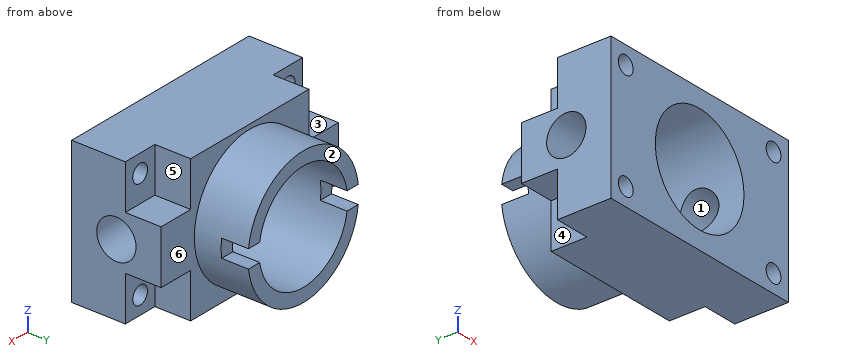
from build123d import *

# Parameters (mm, degrees)
SKETCH_1_W          = 120
SKETCH_1_H          = 80
EXTRUDE_1_DEPTH     = 50
SKETCH_2_W          = 20
SKETCH_2_H          = 25
CUT_EXTRUDE_1_DEPTH = 20
SKETCH_3_R          = 5
CUT_EXTRUDE_2_DEPTH = 30
SKETCH_5_R          = 11
CUT_EXTRUDE_4_DEPTH = 120
SKETCH_6_R          = 37.5
EXTRUDE_2_DEPTH     = 30
SKETCH_7_R          = 30
CUT_EXTRUDE_5_DEPTH = 81
CUT_EXTRUDE_6_DEPTH = 15


with BuildPart() as part:
    # Эскиз1 → Бобышка-Вытянуть1 (new body)
    with BuildSketch(Plane(origin=(0, 0, 0), x_dir=(1, 0, 0), z_dir=(0, 1, 0))):
        Rectangle(SKETCH_1_W, SKETCH_1_H)
    extrude(amount=EXTRUDE_1_DEPTH)

    # Эскиз2 → Вырез-Вытянуть1 (cut)
    with BuildSketch(Plane(origin=(0, 50, 0), x_dir=(1, 0, 0), z_dir=(0, 1, 0))):
        with Locations((-50, 27.5)):
            Rectangle(SKETCH_2_W, SKETCH_2_H)
        with Locations((-50, -27.5)):
            Rectangle(SKETCH_2_W, SKETCH_2_H)
        with Locations((50, -27.5)):
            Rectangle(SKETCH_2_W, SKETCH_2_H)
        with Locations((50, 27.5)):
            Rectangle(SKETCH_2_W, SKETCH_2_H)
    extrude(amount=-CUT_EXTRUDE_1_DEPTH, mode=Mode.SUBTRACT)

    # Эскиз3 → Вырез-Вытянуть2 (cut)
    with BuildSketch(Plane(origin=(0, 30, 0), x_dir=(1, 0, 0), z_dir=(0, 1, 0))):
        with Locations((-50, -30)):
            Circle(SKETCH_3_R)
        with Locations((-50, 30)):
            Circle(SKETCH_3_R)
        with Locations((50, 30)):
            Circle(SKETCH_3_R)
        with Locations((50, -30)):
            Circle(SKETCH_3_R)
    extrude(amount=-CUT_EXTRUDE_2_DEPTH, mode=Mode.SUBTRACT)

    # Эскиз5 → Вырез-Вытянуть4 (cut)
    with BuildSketch(Plane.ZY.offset(60)):
        with Locations((0, 25)):
            Circle(SKETCH_5_R)
    extrude(amount=-CUT_EXTRUDE_4_DEPTH, mode=Mode.SUBTRACT)

    # Эскиз6 → Бобышка-Вытянуть2 (add)
    with BuildSketch(Plane(origin=(0, 50, 0), x_dir=(1, 0, 0), z_dir=(0, 1, 0))):
        Circle(SKETCH_6_R)
    extrude(amount=EXTRUDE_2_DEPTH)

    # Эскиз7 → Вырез-Вытянуть5 (cut, through all)
    with BuildSketch(Plane(origin=(0, 80, 0), x_dir=(1, 0, 0), z_dir=(0, 1, 0))):
        Circle(SKETCH_7_R)
    extrude(amount=-CUT_EXTRUDE_5_DEPTH, mode=Mode.SUBTRACT)

    # Эскиз8 → Вырез-Вытянуть6 (cut)
    with BuildSketch(Plane(origin=(0, 80, 0), x_dir=(1, 0, 0), z_dir=(0, 1, 0))):
        with BuildLine():
            Line((-29.580398915, -5), (-37.165171868, -5))
            ThreePointArc((-37.165171868, -5), (-37.5, 0), (-37.165171868, 5))
            Line((-37.165171868, 5), (-29.580398915, 5))
            ThreePointArc((-29.580398915, 5), (-30, 0), (-29.580398915, -5))
        make_face()
        with BuildLine():
            Line((37.165171868, 5), (29.580398915, 5))
            ThreePointArc((29.580398915, 5), (30, 0), (29.580398915, -5))
            Line((29.580398915, -5), (37.165171868, -5))
            ThreePointArc((37.165171868, -5), (37.5, 0), (37.165171868, 5))
        make_face()
    extrude(amount=-CUT_EXTRUDE_6_DEPTH, mode=Mode.SUBTRACT)


solid = part.part
Model file for the job. Use its own axes, mm. Face numbers are marked on the shaded views. A direction names the side the tool comes from. Give positions to 0.01 mm unless a question says otherwise; leave off trailing zeros. Loops run counter-clockwise (first coordinate to the right, second up) from the corner with the lowest first, then second, coordinate; pieces in that order, holes last. Notation, with made-up numbers: (2, 87.5) -> (11, 87.5) arc R18 ccw to (11, 113.5) -> close; hole circle Ø8 at (45.5, 28.25). An arc over 180 degrees is marked (long way). Use a Markdown table: item, result. Add a question column.
(1) Slice it at D-D on x = 0. List the corners of the cut face in (y, z), and give its area (3 significant figures).
(2) Slice it at A-A on x = 50. List the corners of the cut face in (y, z), and give its area (3 significant figures).
(3) Tool access for the marked faces 4, 5 and 6: list every direction of +Z, -Z, +X, -X, +Y, -Y with a clear straight run to the whole face (end or side of a thin tool).
(4) Wall check: line 1 along X through (y, z) = (29.5, -30.5); line 2 along Z through (x, y) = (-54, 16.5); line 3 along Z through (x, y) = (50, 19.75). Give the ranges that are in metal, low to high.
(5) Slice it at B-B on y = 25. List the corners of the cut face in (x, z), and give its area (3 significant figures).
(6) Mould opens along Y. For the marked faces 1, 2 and 3 say: +Y half, -Y half, draft (parallel to the pull), parting line (faces both ways), or undercut.
(7) Slice it at C-C on z = 19. List the corners of the cut face in (x, y).
(8) Drop flat-ended pins along their axis: pin 1 Ø1.5 at (x, z) = (-24.5, -15.5) entering from -Y; pin 2 Ø8.5 at (x, y) = (32, 73) entering from +Z; pin 3 Ø22 at (x, y) = (55, 37.5) entering from -Z; pin 4 Ø2.5 at (x, z) = (34.5, 0.5) entering from +Y. Give the stop position or say it passes through.
Filled sheet:
| question | item | result |
|---|---|---|
| 1 | outline | (0, -40) -> (50, -40) -> (50, -37.5) -> (80, -37.5) -> (80, -30) -> (0, -30) -> close; (0, 30) -> (80, 30) -> (80, 37.5) -> (50, 37.5) -> (50, 40) -> (0, 40) -> close |
| 1 | area | 1,450 mm2 |
| 2 | outline | (0, -40) -> (30, -40) -> (30, -35) -> (0, -35) -> close; (0, -25) -> (30, -25) -> (30, -15) -> (50, -15) -> (50, 15) -> (30, 15) -> (30, 25) -> (0, 25) -> close; (0, 35) -> (30, 35) -> (30, 40) -> (0, 40) -> close; hole circle Ø22 at (25, 0) |
| 2 | area | 2,020 mm2 |
| 3 | face 4 | -Z, -X, +Y |
| 3 | face 5 | +Z, +X, +Y |
| 3 | face 6 | +Y |
| 4 | line 1 | -60 to -54.97, -45.03 to 45.03, 54.97 to 60 |
| 4 | line 2 | -40 to -33, -27 to -6.98, 6.98 to 27, 33 to 40 |
| 4 | line 3 | -40 to -35, -25 to -9.67, 9.67 to 25, 35 to 40 |
| 5 | outline | (-60, -40) -> (60, -40) -> (60, -11) -> (27.91, -11) arc R30 cw to (-27.91, -11) -> (-60, -11) -> close; (-60, 11) -> (-27.91, 11) arc R30 cw to (27.91, 11) -> (60, 11) -> (60, 40) -> (-60, 40) -> close; hole circle Ø10 at (-50, -30); hole circle Ø10 at (-50, 30); hole circle Ø10 at (50, -30); hole circle Ø10 at (50, 30) |
| 5 | area | 5,110 mm2 |
| 6 | face 1 | undercut |
| 6 | face 2 | +Y half |
| 6 | face 3 | draft |
| 7 | outline | (-60, 0) -> (-23.22, 0) -> (-23.22, 80) -> (-32.33, 80) -> (-32.33, 50) -> (-40, 50) -> (-40, 30) -> (-60, 30) -> close; (23.22, 0) -> (60, 0) -> (60, 30) -> (40, 30) -> (40, 50) -> (32.33, 50) -> (32.33, 80) -> (23.22, 80) -> close |
| 8 | pin 1 | through |
| 8 | pin 2 | z = 25.22 |
| 8 | pin 3 | z = -40 |
| 8 | pin 4 | y = 65 |
